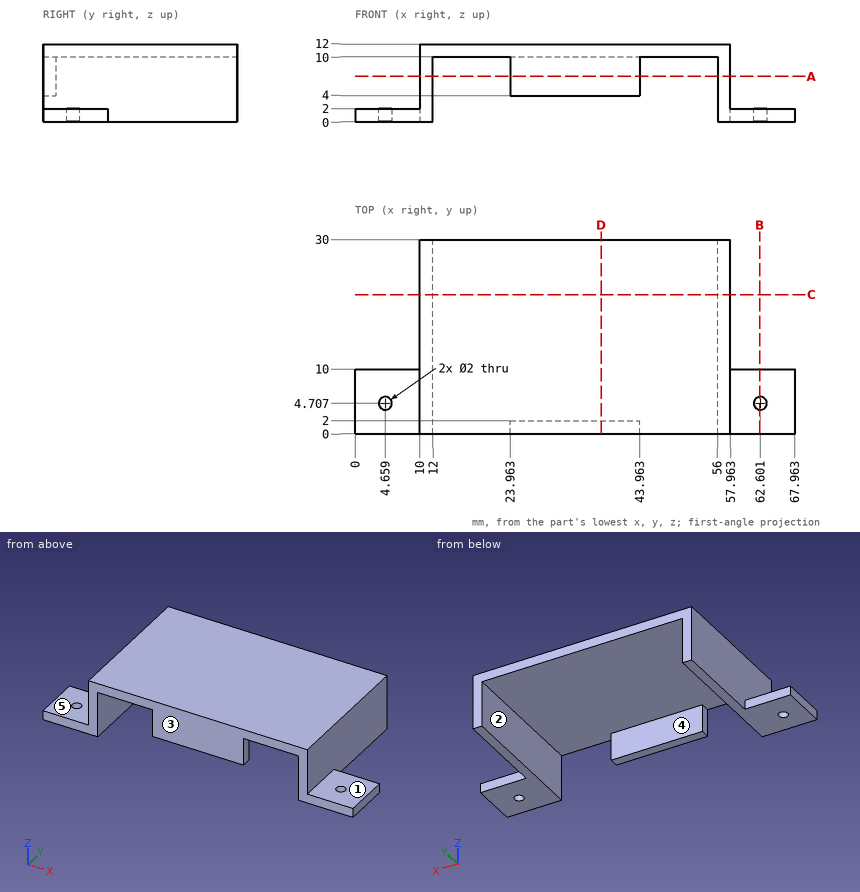
For this review, use the dimensioned drawing (mm, ordinates from the lowest corner) and the shaded views. A direction names the side the tool comes from. Give positions to 0.01 mm unless a question says otherwise; leave off trailing zeros. Order: outer loops, then holes, each group sorted by start corner. A loop starts at its lowest first (then second) coordinate and runs counter-clockwise, first axis right, second up. Notation, with made-up numbers: (2, -7.5) - (34, -7.5) arc R17 cw to (34, 15.5) - close; hole circle Ø2 at (15, -6.75). An arc over 180 degrees is marked (long way). Write item = value, one per line. Start each with the question number.
Q1. We need section A-A on z = 7. State the section outline as (x, y) points, plus the area to 3 significant figures.
Q2. To check wall thickness, follow L1, parallel to X at y = 25.5, z = 6.5; L2, parallel to X at y = 8.25, z = 1.75; L3, parallel to Z at x = 41.5, y = 7.25. State the ranges of each line that lie inside material, in increasing order. Write a range as from..to.
Q3. We need section D-D on x = 38. State the section outline as (y, z) points.
Q4. Mouldability with a two-part tool opening along X and no side actions: class the marked faces 4 and 5 as released by +X, released by -X, zero draft, split by the parting line, or undercut.
Q5. We need section B-B on x = 62.5. State the section outline as (y, z) points.
Q6. Tool access review of the marked faces 1, 2 and 3: name each direction out of +Z, -Z, +X, -X, +Y, -Y from which nothing blocks a thin tool from reaching the whole face with its end or side.
Q7. Clearance check with flat-ended pins moving along their axes: pin 1 Ø1.6 at (x, y) = (4.66, 4.71) entering from +Z; pin 2 Ø0.6 at (x, y) = (38, 1) entering from -Z; pin 3 Ø5 at (x, y) = (62, 5.5) entering from +Z; pin 4 Ø1 at (x, z) = (5, 1.5) entering from +Y. State where each tip first meets the part, or that it passes through.
Q8. We need section C-C on y = 21.5. State the section outline as (x, z) points.
Working result:
q1.outline = (10, 0) - (12, 0) - (12, 30) - (10, 30) - close; (23.96, 0) - (43.96, 0) - (43.96, 2) - (23.96, 2) - close; (56, 0) - (57.96, 0) - (57.96, 30) - (56, 30) - close
q1.area = 159 mm²
q2.L1 = 10..12, 56..57.96
q2.L2 = 0..12, 56..67.96
q2.L3 = 10..12
q3.outline = (0, 4) - (2, 4) - (2, 10) - (30, 10) - (30, 12) - (0, 12) - close
q4.face_4 = undercut
q4.face_5 = zero draft
q5.outline = (0, 0) - (3.71, 0) - (3.71, 2) - (0, 2) - close; (5.7, 0) - (10, 0) - (10, 2) - (5.7, 2) - close
q6.face_1 = +Z, +X, +Y, -Y
q6.face_2 = -Z, +Y, -Y
q6.face_3 = +Z, -Z, +X, -X, -Y
q7.pin_1 = through
q7.pin_2 = 4
q7.pin_3 = 2
q7.pin_4 = 10
q8.outline = (10, 0) - (12, 0) - (12, 10) - (56, 10) - (56, 0) - (57.96, 0) - (57.96, 12) - (10, 12) - close
